from build123d import *

# Parameters (mm, degrees)
SKETCH_1_W          = 439.55
SKETCH_1_H          = 20
SKETCH_1_W_2        = 20
SKETCH_1_H_2        = 170
SKETCH_1_R          = 1.65
EXTRUDE_1_DEPTH     = 5
FILLET_1_R          = 50
FILLET_2_R          = 5
SKETCH_2_R          = 1.5
CUT_EXTRUDE_1_DEPTH = 10
FILLET_3_R          = 10
SKETCH_3_R          = 7.5
CUT_EXTRUDE_2_DEPTH = 10


with BuildPart() as part:
    # ｽｹｯﾁ1 → ﾎﾞｽ - 押し出し1 (new body)
    # profile 1 of 3: a face of its own
    with BuildSketch(Plane.XY):
        with Locations((234.775, 10)):
            Rectangle(SKETCH_1_W, SKETCH_1_H)
    # profile 2 of 3: a face of its own
    with BuildSketch(Plane.XY):
        with Locations((234.775, -10)):
            Rectangle(SKETCH_1_W, SKETCH_1_H)
    # profile 3 of 3: a face of its own
    with BuildSketch(Plane.XY):
        with Locations((5, 0)):
            Rectangle(SKETCH_1_W_2, SKETCH_1_H_2)
        with Locations((10, -80)):
            Circle(SKETCH_1_R, mode=Mode.SUBTRACT)
        with Locations((10, 80)):
            Circle(SKETCH_1_R, mode=Mode.SUBTRACT)
        with Locations((0, 80)):
            Circle(SKETCH_1_R, mode=Mode.SUBTRACT)
        with Locations((0, -80)):
            Circle(SKETCH_1_R, mode=Mode.SUBTRACT)
    extrude(amount=EXTRUDE_1_DEPTH)

    # ﾌｨﾚｯﾄ1
    fillet_1_edges = [part.edges().sort_by_distance(p)[0] for p in [
        (15, 20, 2.5),
        (15, -20, 2.5),
    ]]
    fillet(fillet_1_edges, radius=FILLET_1_R)

    # ﾌｨﾚｯﾄ2
    fillet_2_edges = [part.edges().sort_by_distance(p)[0] for p in [
        (15, -85, 2.5),
        (-5, -85, 2.5),
        (-5, 85, 2.5),
        (15, 85, 2.5),
    ]]
    fillet(fillet_2_edges, radius=FILLET_2_R)

    # ｽｹｯﾁ2 → ｶｯﾄ - 押し出し1 (cut)
    with BuildSketch(Plane.XY.offset(5)):
        with Locations((447.05, 5)):
            Circle(SKETCH_2_R)
        with Locations((447.05, -5)):
            Circle(SKETCH_2_R)
    extrude(amount=-CUT_EXTRUDE_1_DEPTH, mode=Mode.SUBTRACT)

    # ﾌｨﾚｯﾄ3
    fillet_3_edges = [part.edges().sort_by_distance(p)[0] for p in [
        (454.55, 20, 2.5),
        (454.55, -20, 2.5),
    ]]
    fillet(fillet_3_edges, radius=FILLET_3_R)

    # ｽｹｯﾁ3 → ｶｯﾄ - 押し出し2 (cut)
    with BuildSketch(Plane.XY.offset(5)):
        with Locations((15, 0)):
            Circle(SKETCH_3_R)
        with Locations((56.5, 0)):
            Circle(SKETCH_3_R)
        with Locations((98, 0)):
            Circle(SKETCH_3_R)
        with Locations((139.5, 0)):
            Circle(SKETCH_3_R)
        with Locations((181, 0)):
            Circle(SKETCH_3_R)
        with Locations((222.5, 0)):
            Circle(SKETCH_3_R)
        with Locations((264, 0)):
            Circle(SKETCH_3_R)
        with Locations((305.5, 0)):
            Circle(SKETCH_3_R)
        with Locations((347, 0)):
            Circle(SKETCH_3_R)
        with Locations((388.5, 0)):
            Circle(SKETCH_3_R)
        with Locations((430, 0)):
            Circle(SKETCH_3_R)
    extrude(amount=-CUT_EXTRUDE_2_DEPTH, mode=Mode.SUBTRACT)


solid = part.part
Could you check a few things on this model? Use its own coordinates, in mm. Give positions to 0.01 mm unless a question says otherwise; leave off trailing zeros. Loops run counter-clockwise (first coordinate to the right, second up) from the corner with the lowest first, then second, coordinate; pieces in that order, holes last. Notation, with made-up numbers: M 79.25,71.5 L 109.25,71.5 A16 cw 109.25,83.5 Z; hole C 31.25,-12.5 d11. An arc over 180 degrees is marked long. Answer as a JSON object with one key per item and string values.
Q1. Suppose I cut it at A-A, the plane x = 430. List the corners of the cut face in (y, z) for me, plus the area to 3 significant figures.
Values found:
{"outline": "M -20,0 L -7.5,0 L -7.5,5 L -20,5 Z; M 7.5,0 L 20,0 L 20,5 L 7.5,5 Z", "area": "125 mm²"}
Q2. If we mould it in two halves opening along X, with no side actions, what happens to faces 1 (the cylindrical face through (7.507, 0.33, 2.535)), 2 (the flat face through (190, 0, 5)), 3 (the cylindrical face through (29.258, 35.036, 2.535))? For each: pulls with the +X half, pulls with the -X half, needs draft (parallel to the pull), parting line crosses it, or undercut.
Values found:
{"face 1": "undercut", "face 2": "needs draft", "face 3": "pulls with the +X half"}
Q3. Suppose I cut it at B-B, the plane z = 2.1. State how many separate pieces and enclosed holes the cut face has, plus the area to 3 significant figures.
Values found:
{"separate pieces": "1", "enclosed holes": "17", "area": "20,000 mm²"}
Q4. Suppose I cut it at C-C, the plane x = 70. List the corners of the cut face in (y, z) for me.
Values found:
{"outline": "M -20,0 L 20,0 L 20,5 L -20,5 Z"}
Q5. If I drill on probe 1 along X at (y, z) = (-80, 1.45); probe 2 along Y at (x, z) = (0, 2.4); probe 3 along Y at (x, z) = (388.5, 2.3), over which ranges is the centre line in solid material (lowest first)? Write a range as [from, to].
Values found:
{"probe 1": "x = [-5, -1.65], [1.65, 8.35], [11.65, 15]", "probe 2": "y = [-85, -81.65], [-78.35, 78.35], [81.65, 85]", "probe 3": "y = [-20, -7.5], [7.5, 20]"}
Q6. Suppose I cut it at D-D, the plane y = -38. List the corners of the cut face in (x, z) for me.
Values found:
{"outline": "M -5,0 L 26.58,0 L 26.58,5 L -5,5 Z"}
Q7. For P1, Ø2.5, axis at x = 10, y = -80, coming from the +Z side; P2, Ø1.5, axis at y = 75.5, z = 2.5, coming from the +X side; P3, Ø2, axis at y = 53, z = 0.5, coming from the +X side; P4, Ø1.5, axis at x = 310.5, z = 3, coming from the +Y side, each with a flat end and sliding along its axis, tell me the tip position at first contact or that it passes through.
Values found:
{"P1": "passes through", "P2": "stops at x = 15", "P3": "stops at x = 18.35", "P4": "stops at y = 20"}
